Can you work these out from the model? Positions are in its coordinate system, mm. Face numbers are marked on the shaded views. A direction names the side the tool comes from. Coordinates: 2 decimals unless noted, no trailing zeros. Loops run counter-clockwise (first coordinate to the right, second up) from the corner with the lowest first, then second, coordinate; pieces in that order, holes last.
```python
from build123d import *

# Parameters (mm, degrees)
SKETCH2_W           = 63.5
SKETCH2_H           = 88.5
BOSS_EXTRUDE1_DEPTH = 2
SKETCH3_W           = 63.5
SKETCH3_H           = 88.5
SKETCH3_W_2         = 59.5
SKETCH3_H_2         = 84.5
BOSS_EXTRUDE2_DEPTH = 20
SKETCH4_W           = 6.35
SKETCH4_H           = 13
SKETCH4_H_2         = 10.9
CUT_EXTRUDE1_DEPTH  = 2
CHAMFER1_SIZE       = 0.5
SKETCH5_R           = 0.75
SKETCH5_W           = 6.35
SKETCH5_H           = 25
CUT_EXTRUDE3_DEPTH  = 2
FILLET1_R           = 6
SKETCH6_W           = 26.800079737
SKETCH6_H           = 6.35
CUT_EXTRUDE4_DEPTH  = 2
FILLET2_R           = 3
CUT_EXTRUDE5_DEPTH  = 10
BOSS_EXTRUDE3_START = 2
BOSS_EXTRUDE3_DEPTH = 2
SKETCH9_R           = 3.5
SKETCH9_R_2         = 2.5
BOSS_EXTRUDE4_DEPTH = 12.05
SKETCH10_R          = 1.5
CUT_EXTRUDE6_DEPTH  = 76.534322501
SKETCH11_R          = 3
CUT_EXTRUDE7_DEPTH  = 0.5
BOSS_EXTRUDE5_START = 2
SKETCH12_R          = 5
SKETCH12_R_2        = 3
BOSS_EXTRUDE5_DEPTH = 2
CUT_EXTRUDE8_DEPTH  = 3


with BuildPart() as part:
    # Sketch2 → Boss-Extrude1 (new body)
    with BuildSketch(Plane.XY.offset(2)):
        with Locations((-8.071244, 16.046786)):
            Rectangle(SKETCH2_W, SKETCH2_H)
    extrude(amount=BOSS_EXTRUDE1_DEPTH)

    # Sketch3 → Boss-Extrude2 (add)
    with BuildSketch(Plane(origin=(0, 0, 2), x_dir=(-1, 0, 0), z_dir=(0, 0, -1))):
        with Locations((8.071244, 16.046786)):
            Rectangle(SKETCH3_W, SKETCH3_H)
        with Locations((8.071244, 16.046786)):
            Rectangle(SKETCH3_W_2, SKETCH3_H_2, mode=Mode.SUBTRACT)
    extrude(amount=BOSS_EXTRUDE2_DEPTH)

    # Sketch4 → Cut-Extrude1 (cut)
    with BuildSketch(Plane(origin=(23.678756, 0, 0), x_dir=(0, 0, -1), z_dir=(1, 0, 0))):
        with Locations((14.825, 35.546786)):
            Rectangle(SKETCH4_W, SKETCH4_H)
        with Locations((14.825, 49.296786)):
            Rectangle(SKETCH4_W, SKETCH4_H_2)
    extrude(amount=-CUT_EXTRUDE1_DEPTH, mode=Mode.SUBTRACT)

    # Chamfer1
    chamfer1_edges = [part.edges().sort_by_distance(p)[0] for p in [
        (23.678756, 42.046786, -14.825),
        (23.678756, 35.546786, -11.65),
        (23.678756, 29.046786, -14.825),
        (23.678756, 54.746786, -14.825),
        (23.678756, 49.296786, -11.65),
        (23.678756, 43.846786, -14.825),
    ]]
    chamfer(chamfer1_edges, length=CHAMFER1_SIZE)

    # Sketch5 → Cut-Extrude3 (cut)
    with BuildSketch(Plane.ZY.offset(39.821244)):
        with Locations(Location((-12.431991388, 40.654286, 0), (0, 0, 270))):
            Circle(SKETCH5_R)
        with Locations((-14.825, 21.706977335)):
            Rectangle(SKETCH5_W, SKETCH5_H)
    extrude(amount=-CUT_EXTRUDE3_DEPTH, mode=Mode.SUBTRACT)

    # Fillet1
    fillet1_edges = [part.edges().sort_by_distance(p)[0] for p in [
        (-38.821244, 34.206977335, -18),
        (-38.821244, 9.206977335, -18),
    ]]
    fillet(fillet1_edges, radius=FILLET1_R)

    # Sketch6 → Cut-Extrude4 (cut)
    with BuildSketch(Plane.XZ.offset(28.203214)):
        with Locations((-0.390288681, -14.825)):
            Rectangle(SKETCH6_W, SKETCH6_H)
    extrude(amount=-CUT_EXTRUDE4_DEPTH, mode=Mode.SUBTRACT)

    # Fillet2
    fillet2_edges = [part.edges().sort_by_distance(p)[0] for p in [
        (-39.821244, 60.296786, -7),
        (23.678756, 60.296786, -7),
        (23.678756, -28.203214, -7),
        (-39.821244, -28.203214, -7),
    ]]
    fillet(fillet2_edges, radius=FILLET2_R)

    # Sketch7 → Cut-Extrude5 (cut)
    with BuildSketch(Plane.XY.offset(4)):
        with BuildLine():
            Line((-2.571244, -10.203214), (-5.198962677, -10.203214))
            ThreePointArc((-5.198962677, -10.203214), (-8.071244, -11.703214), (-10.943525323, -10.203214))
            Line((-10.943525323, -10.203214), (-13.571244, -10.203214))
            ThreePointArc((-13.571244, -10.203214), (-15.571244, -8.203214), (-13.571244, -6.203214))
            Line((-13.571244, -6.203214), (-10.943525323, -6.203214))
            ThreePointArc((-10.943525323, -6.203214), (-10.546117734, -5.728340266), (-10.071244, -5.330932677))
            Line((-10.071244, -5.330932677), (-10.071244, -2.703214))
            ThreePointArc((-10.071244, -2.703214), (-8.071244, -0.703214), (-6.071244, -2.703214))
            Line((-6.071244, -2.703214), (-6.071244, -5.330932677))
            ThreePointArc((-6.071244, -5.330932677), (-5.596370266, -5.728340266), (-5.198962677, -6.203214))
            Line((-5.198962677, -6.203214), (-2.571244, -6.203214))
            ThreePointArc((-2.571244, -6.203214), (-0.571244, -8.203214), (-2.571244, -10.203214))
        make_face()
        with BuildLine():
            Line((-6.071244, 34.796786), (-6.071244, 37.424504677))
            ThreePointArc((-6.071244, 37.424504677), (-5.596370266, 37.821912266), (-5.198962677, 38.296786))
            Line((-5.198962677, 38.296786), (-2.571244, 38.296786))
            ThreePointArc((-2.571244, 38.296786), (-0.571244, 40.296786), (-2.571244, 42.296786))
            Line((-2.571244, 42.296786), (-5.198962677, 42.296786))
            ThreePointArc((-5.198962677, 42.296786), (-8.071244, 43.796786), (-10.943525323, 42.296786))
            Line((-10.943525323, 42.296786), (-13.571244, 42.296786))
            ThreePointArc((-13.571244, 42.296786), (-15.571244, 40.296786), (-13.571244, 38.296786))
            Line((-13.571244, 38.296786), (-10.943525323, 38.296786))
            ThreePointArc((-10.943525323, 38.296786), (-10.546117734, 37.821912266), (-10.071244, 37.424504677))
            Line((-10.071244, 37.424504677), (-10.071244, 34.796786))
            ThreePointArc((-10.071244, 34.796786), (-8.071244, 32.796786), (-6.071244, 34.796786))
        make_face()
    extrude(amount=-CUT_EXTRUDE5_DEPTH, mode=Mode.SUBTRACT)

    # Sketch8 → Boss-Extrude3 (add)
    with BuildSketch(Plane.XY.offset(4).offset(BOSS_EXTRUDE3_START)):
        with BuildLine():
            Line((-11.846161218, 44.296786), (-13.571244, 44.296786))
            ThreePointArc((-13.571244, 44.296786), (-17.571244, 40.296786), (-13.571244, 36.296786))
            Line((-13.571244, 36.296786), (-12.071244, 36.296786))
            Line((-12.071244, 36.296786), (-12.071244, 34.796786))
            ThreePointArc((-12.071244, 34.796786), (-8.071244, 30.796786), (-4.071244, 34.796786))
            Line((-4.071244, 34.796786), (-4.071244, 36.296786))
            Line((-4.071244, 36.296786), (-2.571244, 36.296786))
            ThreePointArc((-2.571244, 36.296786), (1.428756, 40.296786), (-2.571244, 44.296786))
            Line((-2.571244, 44.296786), (-4.296326782, 44.296786))
            ThreePointArc((-4.296326782, 44.296786), (-8.071244, 45.796786), (-11.846161218, 44.296786))
        make_face()
        with BuildLine():
            Line((-2.571244, 42.296786), (-5.198962677, 42.296786))
            ThreePointArc((-5.198962677, 42.296786), (-8.071244, 43.796786), (-10.943525323, 42.296786))
            Line((-10.943525323, 42.296786), (-13.571244, 42.296786))
            ThreePointArc((-13.571244, 42.296786), (-15.571244, 40.296786), (-13.571244, 38.296786))
            Line((-13.571244, 38.296786), (-10.943525323, 38.296786))
            ThreePointArc((-10.943525323, 38.296786), (-10.546117734, 37.821912266), (-10.071244, 37.424504677))
            Line((-10.071244, 37.424504677), (-10.071244, 34.796786))
            ThreePointArc((-10.071244, 34.796786), (-8.071244, 32.796786), (-6.071244, 34.796786))
            Line((-6.071244, 34.796786), (-6.071244, 37.424504677))
            ThreePointArc((-6.071244, 37.424504677), (-5.596370266, 37.821912266), (-5.198962677, 38.296786))
            Line((-5.198962677, 38.296786), (-2.571244, 38.296786))
            ThreePointArc((-2.571244, 38.296786), (-0.571244, 40.296786), (-2.571244, 42.296786))
        make_face(mode=Mode.SUBTRACT)
    boss_extrude3 = extrude(amount=-BOSS_EXTRUDE3_DEPTH)

    # Sketch9 → Boss-Extrude4 (add)
    with BuildSketch(Plane(origin=(0, 0, 2), x_dir=(-1, 0, 0), z_dir=(0, 0, -1))):
        with Locations(Location((-15.678756, -20.703214, 0), (0, 0, 180))):
            Circle(SKETCH9_R)
        with Locations(Location((32.321244, 5.296786, 0), (0, 0, 180))):
            Circle(SKETCH9_R)
        with Locations(Location((-7.678756, 53.796786, 0), (0, 0, 180))):
            Circle(SKETCH9_R_2)
    extrude(amount=BOSS_EXTRUDE4_DEPTH)

    # Sketch10 → Cut-Extrude6 (cut, through all)
    with BuildSketch(Plane.XY.offset(4)):
        with Locations((7.678756, 53.796786)):
            Circle(SKETCH10_R)
        with Locations((15.678756, -20.703214)):
            Circle(SKETCH10_R)
        with Locations((-32.321244, 5.296786)):
            Circle(SKETCH10_R)
    extrude(amount=-CUT_EXTRUDE6_DEPTH, mode=Mode.SUBTRACT)

    # Sketch11 → Cut-Extrude7 (cut)
    with BuildSketch(Plane.XY.offset(4)):
        with Locations((7.678756, 53.796786)):
            Circle(SKETCH11_R)
        with Locations((-32.321244, 5.296786)):
            Circle(SKETCH11_R)
        with Locations((15.678756, -20.703214)):
            Circle(SKETCH11_R)
    extrude(amount=-CUT_EXTRUDE7_DEPTH, mode=Mode.SUBTRACT)

    # Sketch12 → Boss-Extrude5 (add)
    # profile 1 of 3: a face of its own
    with BuildSketch(Plane.XY.offset(4).offset(BOSS_EXTRUDE5_START)):
        with Locations((7.678756, 53.796786)):
            Circle(SKETCH12_R)
        with Locations((7.678756, 53.796786)):
            Circle(SKETCH12_R_2, mode=Mode.SUBTRACT)
    # profile 2 of 3: a face of its own
    with BuildSketch(Plane.XY.offset(4).offset(BOSS_EXTRUDE5_START)):
        with Locations((-32.321244, 5.296786)):
            Circle(SKETCH12_R)
        with Locations((-32.321244, 5.296786)):
            Circle(SKETCH12_R_2, mode=Mode.SUBTRACT)
    # profile 3 of 3: a face of its own
    with BuildSketch(Plane.XY.offset(4).offset(BOSS_EXTRUDE5_START)):
        with Locations((15.678756, -20.703214)):
            Circle(SKETCH12_R)
        with Locations((15.678756, -20.703214)):
            Circle(SKETCH12_R_2, mode=Mode.SUBTRACT)
    extrude(amount=-BOSS_EXTRUDE5_DEPTH)

    # Sketch13 → Cut-Extrude8 (cut)
    with BuildSketch(Plane(origin=(0, 0, 2), x_dir=(-1, 0, 0), z_dir=(0, 0, -1))):
        with BuildLine():
            Line((13.571244, 43.296786), (11.425345966, 43.296786))
            ThreePointArc((11.425345966, 43.296786), (8.071244, 44.796786), (4.717142034, 43.296786))
            Line((4.717142034, 43.296786), (2.571244, 43.296786))
            ThreePointArc((2.571244, 43.296786), (-0.428756, 40.296786), (2.571244, 37.296786))
            Line((2.571244, 37.296786), (4.717142034, 37.296786))
            ThreePointArc((4.717142034, 37.296786), (4.889263485, 37.114805485), (5.071244, 36.942684034))
            Line((5.071244, 36.942684034), (5.071244, 34.796786))
            ThreePointArc((5.071244, 34.796786), (8.071244, 31.796786), (11.071244, 34.796786))
            Line((11.071244, 34.796786), (11.071244, 36.942684034))
            ThreePointArc((11.071244, 36.942684034), (11.253224515, 37.114805485), (11.425345966, 37.296786))
            Line((11.425345966, 37.296786), (13.571244, 37.296786))
            ThreePointArc((13.571244, 37.296786), (16.571244, 40.296786), (13.571244, 43.296786))
        make_face()
    cut_extrude8 = extrude(amount=-CUT_EXTRUDE8_DEPTH, mode=Mode.SUBTRACT)

    # Mirror1: Boss-Extrude3, Cut-Extrude8 across plane
    add(boss_extrude3.mirror(Plane.ZX.offset(16.046786)))
    add(cut_extrude8.mirror(Plane.ZX.offset(16.046786)), mode=Mode.SUBTRACT)


solid = part.part
```
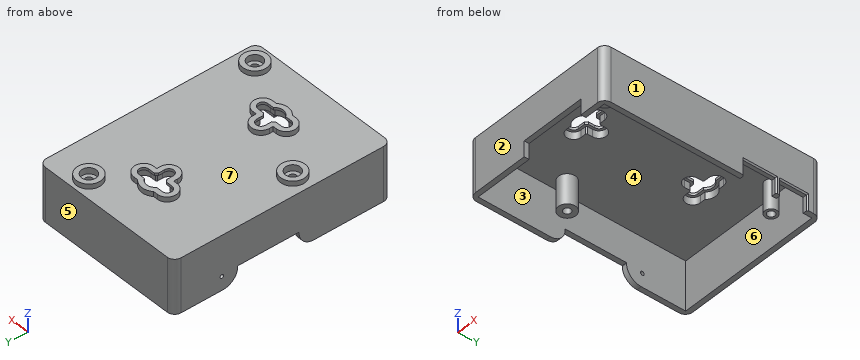
(1) I want a section at A-A on y = 20.5. Write out the boundary of the cut face in (x, z), then the cut area to 3 significant figures.
Check values:
outline: (-39.82, -11.65) - (-37.82, -11.65) - (-37.82, 2) - (21.68, 2) - (21.68, -18) - (23.68, -18) - (23.68, 4) - (-39.82, 4) - close
area: 194 mm2
(2) I want a section at C-C on y = -7.5. Write out the boundary of the cut face in (x, z).
Check values:
outline: (-39.82, -18) - (-37.82, -18) - (-37.82, 2) - (-16.49, 2) - (-16.49, 5) - (-15.44, 5) - (-15.44, 6) - (-17.51, 6) - (-17.51, 4) - (-39.82, 4) - close; (-0.7, 5) - (0.35, 5) - (0.35, 2) - (21.68, 2) - (21.68, -18) - (23.68, -18) - (23.68, 4) - (1.37, 4) - (1.37, 6) - (-0.7, 6) - close
(3) I'm going to push flat-ended pins straight in: pin 1 (5 mm diameter, centred on x = 16.5, y = 10.5, fed in from -Z); pin 2 (0.6 mm diameter, centred on y = -27.5, z = -14.5, fed in from -X); pin 3 (5 mm diameter, centred on x = 15.68, y = -20.7, fed in from -Z). Where does each tip first touch, or does it pass through?
Check values:
pin 1: stops at z = 2
pin 2: stops at x = -39.06
pin 3: stops at z = -10.05
(4) If we mould it in two halves opening along Y, with no side actions, what happens to the marked faces 1, 2, 3 and 4? For each: released by +Y, released by -Y, zero draft, split by the parting line, or undercut.
Check values:
face 1: zero draft
face 2: released by -Y
face 3: undercut
face 4: undercut
(5) I want a section at D-D on x = -7. State how many separate pieces and enclosed holes the cut face has, then the cut area to 3 significant figures.
Check values:
separate pieces: 3
enclosed holes: 0
area: 206 mm2
(6) If I drill on probe 1 along Y at (x, z) = (8, -10.5); probe 2 along X at (y, z) = (39.5, -7.25); probe 3 along X at (y, z) = (-23.5, 0.5), over which ranges is the centre line in solid material (lowest first)?
Check values:
probe 1: y = -28.2 to -26.2, 58.3 to 60.3
probe 2: x = -39.82 to -37.82, 21.68 to 23.68
probe 3: x = -39.82 to -37.82, 13.57 to 17.78, 21.68 to 23.68
(7) Which directions (+Z, -Z, +X, -X, +Y, -Y) give clear straight access to the entire face, cutting with the end or side of a thin tool? Please do the marked faces 5, 6 and 7.
Check values:
face 5: +Z, -Z, +X, -X, +Y
face 6: -Z
face 7: +Z
(8) I want a section at B-B on z = -7.25. Write out the boundary of the cut face in (x, y).
Check values:
outline: (-39.82, -25.2) arc R3 ccw to (-36.82, -28.2) - (20.68, -28.2) arc R3 ccw to (23.68, -25.2) - (23.68, 57.3) arc R3 ccw to (20.68, 60.3) - (-36.82, 60.3) arc R3 ccw to (-39.82, 57.3) - close; circle Ø7 at (-32.32, 5.3); circle Ø5 at (7.68, 53.8); circle Ø7 at (15.68, -20.7); hole (-37.82, -26.2) - (21.68, -26.2) - (21.68, 58.3) - (-37.82, 58.3) - close; hole circle Ø3 at (-32.32, 5.3); hole circle Ø3 at (7.68, 53.8); hole circle Ø3 at (15.68, -20.7)
